```python
from build123d import *

# Parameters (mm, degrees)
BOSS_EXTRUDE1_START                             = -18.668682
BOSS_EXTRUDE1_OUTLINE_R                         = 49
BOSS_EXTRUDE1_DEPTH                             = 18.668682
BOSS_EXTRUDE1_START_2                           = -56
BOSS_EXTRUDE1_2_OUTLINE_R                       = 49
BOSS_EXTRUDE1_2_OUTLINE_R_2                     = 45
BOSS_EXTRUDE1_2_DEPTH                           = 37.331318
BOSS_EXTRUDE1_START_3                           = -4
BOSS_EXTRUDE1_3_OUTLINE_R                       = 60.625
BOSS_EXTRUDE1_3_OUTLINE_R_2                     = 49
BOSS_EXTRUDE1_3_DEPTH                           = 4
BOSS_EXTRUDE1_START_4                           = -13
BOSS_EXTRUDE1_4_DEPTH                           = 26
CUT_EXTRUDE1_DEPTH                              = 1.918682
CUT_EXTRUDE2_REACH                              = 112.599
CUT_EXTRUDE3_DEPTH                              = 103.404986
CUT_EXTRUDE4_DEPTH                              = 103.404986
CUT_EXTRUDE5_DEPTH                              = 12.75
CUT_EXTRUDE6_DEPTH                              = 18
SKETCH16_W                                      = 8
SKETCH16_H                                      = 26
BOSS_EXTRUDE2_DEPTH                             = 34
CUT_EXTRUDE7_DEPTH                              = 101.273532
CUT_EXTRUDE8_REACH                              = 111.441
SKETCH23_W                                      = 10
SKETCH23_H                                      = 24
F_3_4_3_4_DIAMETER_HOLE1_D                      = 3.4
SKETCH26_W                                      = 5
SKETCH26_H                                      = 105.34636
F_2_6_2_6_DIAMETER_HOLE1_D                      = 2.6
F_2_6_2_6_DIAMETER_HOLE1_DEPTH                  = 7.2
CSK_FOR_M3_FLAT_HEAD_MACHINE_SCREW1_D           = 3.4
CSK_FOR_M3_FLAT_HEAD_MACHINE_SCREW1_DEPTH       = 30.178537
CSK_FOR_M3_FLAT_HEAD_MACHINE_SCREW1_CSINK_D     = 6.3
CSK_FOR_M3_FLAT_HEAD_MACHINE_SCREW1_CSINK_ANGLE = 90
CSK_FOR_M3_FLAT_HEAD_MACHINE_SCREW1_TIP         = 1.021463


with BuildPart() as part:
    # Boss-Extrude1: read off the stored shape, not the designer's step
    # Boss-Extrude1 outline → Boss-Extrude1 (new body)
    with BuildSketch(Plane.XZ.offset(BOSS_EXTRUDE1_START)):
        Circle(BOSS_EXTRUDE1_OUTLINE_R)
        with BuildLine():
            Line((-10.445584, 13), (29.067401, -34.352383))
            ThreePointArc((29.067401, -34.352383), (-34.551051, -28.830971), (-28.593183, 34.748092))
            Line((-28.593183, 34.748092), (-10.445584, 13))
        make_face(mode=Mode.SUBTRACT)
    extrude(amount=BOSS_EXTRUDE1_DEPTH)

    # Boss-Extrude1 2 outline → Boss-Extrude1 2 (add)
    with BuildSketch(Plane.XZ.offset(BOSS_EXTRUDE1_START_2)):
        Circle(BOSS_EXTRUDE1_2_OUTLINE_R)
        Circle(BOSS_EXTRUDE1_2_OUTLINE_R_2, mode=Mode.SUBTRACT)
    extrude(amount=BOSS_EXTRUDE1_2_DEPTH)

    # Boss-Extrude1 3 outline → Boss-Extrude1 3 (add)
    with BuildSketch(Plane.XZ.offset(BOSS_EXTRUDE1_START_3)):
        Circle(BOSS_EXTRUDE1_3_OUTLINE_R)
        Circle(BOSS_EXTRUDE1_3_OUTLINE_R_2, mode=Mode.SUBTRACT)
    extrude(amount=BOSS_EXTRUDE1_3_DEPTH)

    # Boss-Extrude1 4 outline → Boss-Extrude1 4 (add)
    with BuildSketch(Plane.XY.offset(BOSS_EXTRUDE1_START_4)):
        Polygon((-46.75, 15), (-5.75, 56), (-47, 56), (-47, 15), align=None)
    extrude(amount=BOSS_EXTRUDE1_4_DEPTH)

    # Sketch2 → Cut-Extrude1 (cut)
    with BuildSketch(Plane(origin=(0, 18.668682, 0), x_dir=(-1, 0, 0), z_dir=(0, 1, 0))):
        with BuildLine():
            Line((-29.067401, -34.352383), (28.593183, 34.748092))
            ThreePointArc((28.593183, 34.748092), (-34.551051, 28.830971), (-29.067401, -34.352383))
        make_face()
    extrude(amount=-CUT_EXTRUDE1_DEPTH, mode=Mode.SUBTRACT)

    # Sketch7 → Cut-Extrude2 (cut, up to next)
    with BuildSketch(Plane.XY.offset(13), mode=Mode.PRIVATE) as cut_extrude2_sk1:
        Polygon((-31.75, 56), (-31.75, 30), (-5.75, 56), align=None)
    cut_extrude2_tool1 = extrude(cut_extrude2_sk1.sketch, amount=-CUT_EXTRUDE2_REACH, mode=Mode.PRIVATE) & part.part
    add(cut_extrude2_tool1.solids().sort_by_distance((-23.083333, 47.333333, 13))[0], mode=Mode.SUBTRACT)

    # Sketch12 → Cut-Extrude3 (cut, through all)
    with BuildSketch(Plane.XZ):
        with BuildLine():
            Line((-28.593183, 34.748092), (0.402208, 0))
            Line((0.402208, 0), (29.067401, 34.352383))
            ThreePointArc((29.067401, 34.352383), (0.308816, 44.99894), (-28.593183, 34.748092))
        make_face()
    extrude(amount=-CUT_EXTRUDE3_DEPTH, mode=Mode.SUBTRACT)

    # Sketch13 → Cut-Extrude4 (cut, through all)
    with BuildSketch(Plane.XZ):
        Polygon((0.402208, 0), (11.25, -13), (11.25, 13), align=None)
    extrude(amount=-CUT_EXTRUDE4_DEPTH, mode=Mode.SUBTRACT)

    # Sketch14 → Cut-Extrude5 (cut)
    with BuildSketch(Plane(origin=(0, 16.75, 0), x_dir=(-1, 0, 0), z_dir=(0, 1, 0))):
        with BuildLine():
            Line((-11.25, -13), (-11.25, 13))
            Line((-11.25, 13), (-29.067401, 34.352383))
            ThreePointArc((-29.067401, 34.352383), (-45, 0), (-29.067401, -34.352383))
            Line((-29.067401, -34.352383), (-11.25, -13))
        make_face()
    extrude(amount=-CUT_EXTRUDE5_DEPTH, mode=Mode.SUBTRACT)

    # Sketch15 → Cut-Extrude6 (cut)
    with BuildSketch(Plane(origin=(0, 56, 0), x_dir=(-1, 0, 0), z_dir=(0, 1, 0))):
        with BuildLine():
            Line((43.081318, 13), (31.75, 13))
            Line((31.75, 13), (31.75, -13))
            Line((31.75, -13), (43.081318, -13))
            ThreePointArc((43.081318, -13), (45, 0), (43.081318, 13))
        make_face()
    extrude(amount=-CUT_EXTRUDE6_DEPTH, mode=Mode.SUBTRACT)

    # Sketch16 → Boss-Extrude2 (add)
    with BuildSketch(Plane(origin=(0, 4, 0), x_dir=(-1, 0, 0), z_dir=(0, 1, 0))):
        with Locations((-15.25, 0)):
            Rectangle(SKETCH16_W, SKETCH16_H)
    extrude(amount=BOSS_EXTRUDE2_DEPTH)

    # Sketch17 → Cut-Extrude7 (cut, through all)
    with BuildSketch(Plane(origin=(0, 4, 0), x_dir=(-1, 0, 0), z_dir=(0, 1, 0))):
        with BuildLine():
            Line((-29.479537, -22.359715), (-24.25, -16.092635))
            Line((-24.25, -16.092635), (-24.25, 16.092635))
            Line((-24.25, 16.092635), (-29.479537, 22.359715))
            ThreePointArc((-29.479537, 22.359715), (-37, 0), (-29.479537, -22.359715))
        make_face()
    extrude(amount=-CUT_EXTRUDE7_DEPTH, mode=Mode.SUBTRACT)

    # Sketch23 → Cut-Extrude8 (cut, up to next)
    with BuildSketch(Plane.ZY.offset(-11.25), mode=Mode.PRIVATE) as cut_extrude8_sk1:
        with Locations((0, 17)):
            Rectangle(SKETCH23_W, SKETCH23_H)
    cut_extrude8_tool1 = extrude(cut_extrude8_sk1.sketch, amount=-CUT_EXTRUDE8_REACH, mode=Mode.PRIVATE) & part.part
    add(cut_extrude8_tool1.solids().sort_by_distance((11.25, 17, 0))[0], mode=Mode.SUBTRACT)

    # Ø3.4 (3.4) Diameter Hole1 (through all)
    with Locations(Plane(origin=(0, 4, 0), x_dir=(1, 0, 0), z_dir=(0, 1, 0))):
        with Locations((38.890873, 38.890873), (38.890873, -38.890873), (-38.890873, -38.890873), (-38.890873, 38.890873)):
            Hole(F_3_4_3_4_DIAMETER_HOLE1_D / 2)

    # Sketch26 → Ø10.0 (10) Diameter Hole1 (revolve, cut)
    with BuildSketch(Plane(origin=(44.72136, 14, 0), x_dir=(0, 0, -1), z_dir=(0, 1, 0))):
        with Locations((2.5, 52.67318)):
            Rectangle(SKETCH26_W, SKETCH26_H)
    revolve(axis=Axis((51.07136, 14, 0), (-1, 0, 0)), mode=Mode.SUBTRACT)

    # Ø2.6 (2.6) Diameter Hole1
    with Locations(Plane(origin=(0, 38, 0), x_dir=(1, 0, 0), z_dir=(0, 1, 0))):
        with Locations((13.75, -5), (13.75, 5), (-34.25, 5), (-34.25, -5)):
            Hole(F_2_6_2_6_DIAMETER_HOLE1_D / 2, depth=F_2_6_2_6_DIAMETER_HOLE1_DEPTH)

    # CSK for M3 Flat Head Machine Screw1
    with Locations(Plane(origin=(0, 56, 0), x_dir=(1, 0, 0), z_dir=(0, 1, 0))):
        with Locations((0, 47), (-47, 0), (-0.090425, -46.999913), (46.999978, -0.045213)):
            CounterSinkHole(CSK_FOR_M3_FLAT_HEAD_MACHINE_SCREW1_D / 2, CSK_FOR_M3_FLAT_HEAD_MACHINE_SCREW1_CSINK_D / 2, depth=CSK_FOR_M3_FLAT_HEAD_MACHINE_SCREW1_DEPTH, counter_sink_angle=CSK_FOR_M3_FLAT_HEAD_MACHINE_SCREW1_CSINK_ANGLE)
            with Locations((0, 0, -(CSK_FOR_M3_FLAT_HEAD_MACHINE_SCREW1_DEPTH + CSK_FOR_M3_FLAT_HEAD_MACHINE_SCREW1_TIP / 2))):  # 118° drill point
                Cone(0, CSK_FOR_M3_FLAT_HEAD_MACHINE_SCREW1_D / 2, CSK_FOR_M3_FLAT_HEAD_MACHINE_SCREW1_TIP, mode=Mode.SUBTRACT)


solid = part.part
```
Design review of the part built by this model. Coordinates are the model's own, in mm. A direction names the side the tool comes from. Give positions to 0.01 mm unless a question says otherwise; leave off trailing zeros. Loops run counter-clockwise (first coordinate to the right, second up) from the corner with the lowest first, then second, coordinate; pieces in that order, holes last. Notation, with made-up numbers: M 71,-23 L 127,-23 A11 ccw 127,-19 Z; hole C 33,1 d1. An arc over 180 degrees is marked long. Return JSON: item names as keys, results as strings. Group by question number.
Item 1: We need section A-A (x = -12.5). Give the boundary of the cut face in (y, z), and give its area (3 significant figures).
Item 2: Mouldability with a two-part tool opening along Z and no side actions: class faces 5 (the flat face through (15, 29, 0)), 6 (the flat face through (-33, 56, -32)) as released by +Z, released by -Z, zero draft, split by the parting line, or undercut.
Item 3: Tool access review of faces 1 (the flat face through (-31, 56, 33)), 2 (the flat face through (20.034, 1.972, 23.527)), 3 (the flat face through (-5, 4, -49)), 4 (the flat face through (15, 17, 5)): name each direction out of +Z, -Z, +X, -X, +Y, -Y from which nothing blocks a thin tool from reaching the whole face with its end or side.
Item 4: Insertion check: pin 1 Ø9 at (x, y) = (15.5, 24.5) entering from -Z; pin 2 Ø1 at (y, z) = (34.5, -0.5) entering from -X; pin 3 Ø1.5 at (y, z) = (8, -5) entering from -X. Each pin has a flat end and moves straight along its axis. Give the tip position at first contact, or say it passes through.
Item 5: We need section D-D (x = -51.5). Give the boundary of the cut face in (y, z), and give its area (3 significant figures).
Item 6: We need section C-C (y = 49). Give the boundary of the cut face in (x, z).
Item 7: For probe 1 along Z at (x, y) = (0, 47); probe 2 along Z at (x, y) = (-1.5, 15.5) (3 decimals); probe 3 along Z at (x, y) = (13, 34), list the stretches that pass through material, from the lowest coordinate up.
Item 8: We need section B-B (y = 10.5). Give the boundary of the cut face in (x, z).
Output:
{
 "1": {"outline": "M 0,-59.32 L 4,-59.32 L 4,-47.38 L 56,-47.38 L 56,-43.23 L 0,-43.23 Z; M 0,43.23 L 56,43.23 L 56,47.38 L 4,47.38 L 4,59.32 L 0,59.32 Z", "area": "560 mm^2"},
 "2": {"face 5": "undercut", "face 6": "zero draft"},
 "3": {"face 1": "+Z, -Z, +X, -X, +Y", "face 2": "+Y, -Y", "face 3": "+Y", "face 4": "none"},
 "4": {"pin 1": "stops at z = -47.75", "pin 2": "stops at x = -49", "pin 3": "stops at x = -48.82"},
 "5": {"outline": "M 0,-31.99 L 4,-31.99 L 4,31.99 L 0,31.99 Z", "area": "256 mm^2"},
 "6": {"outline": "C 0,0 d98; hole C -47,0 d3.4; hole M -43.08,-13 A45 ccw long -43.08,13 A45 ccw Z; hole C -0.09,47 d3.4; hole C 0,-47 d3.4; hole C 47,0.05 d3.4"},
 "7": {"probe 1": "z = -49 to -48.7, -45.3 to -45, 45 to 45.3, 48.7 to 49", "probe 2": "z = -48.977 to -44.975, 44.975 to 48.977", "probe 3": "z = -47.24 to -43.08, -13 to -6.06, -3.94 to 3.94, 6.06 to 13, 43.08 to 47.24"},
 "8": {"outline": "M -48.87,-3.57 A49 ccw long -48.87,3.57 L -44.86,3.57 A45 cw -28.59,34.75 A45 cw 29.07,34.35 A45 cw long -44.86,-3.57 Z; M 11.25,-13 L 19.25,-13 L 19.25,-5 L 11.25,-5 Z; M 11.25,5 L 19.25,5 L 19.25,13 L 11.25,13 Z"}
}
